Geometry: see drawing. Coordinates: mm, zero at the bounding-box minimum. Coordinates: 2 decimals unless noted, no trailing zeros. Loops run counter-clockwise (first coordinate to the right, second up) from the corner with the lowest first, then second, coordinate; pieces in that order, holes last. Notation, with made-up numbers: (-21.5, 53) -> (-4.5, 53) arc R27 ccw to (-4.5, 70) -> close; hole circle Ø7 at (45.25, 3.5). An arc over 180 degrees is marked (long way). One line per item, written item: value. Start each with the question number.
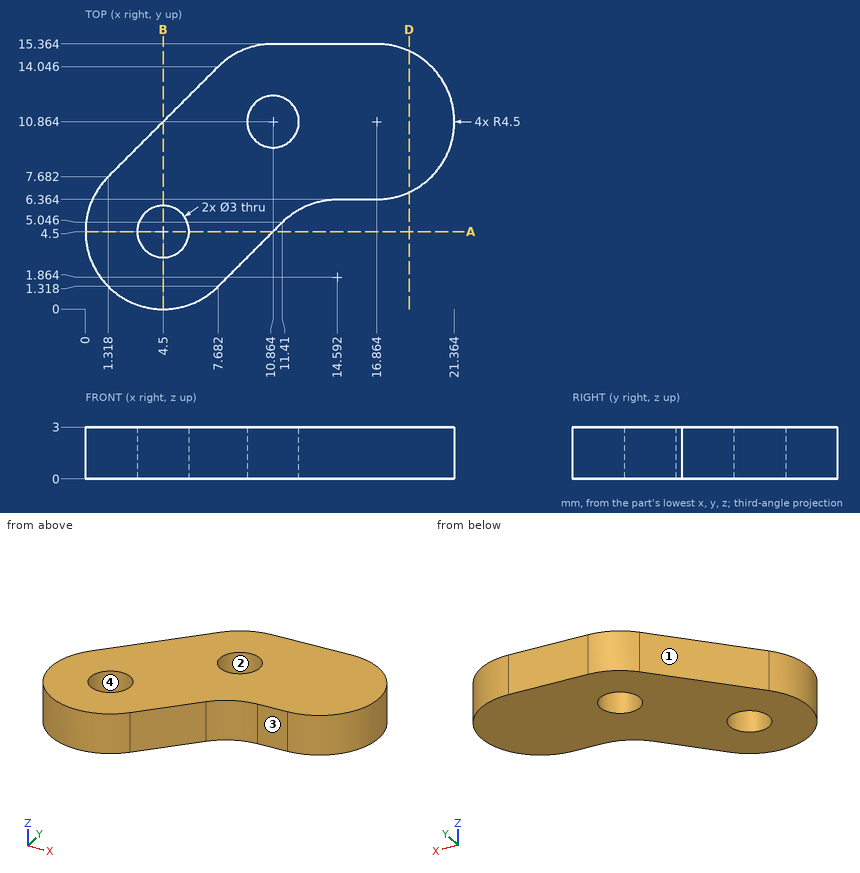
1. Draft query along Y for the marked faces 1, 2, 3 and 4. Return one class per face: released by +Y, released by -Y, zero draft, split by the parting line, or undercut.
2. Section A-A on y = 4.5. Return the cut outline in (x, z), plus the area to 3 significant figures.
3. Section D-D on x = 18.75. Return the cut outline in (y, z), plus the area to 3 significant figures.
4. Pin query (flat end, axial travel): pin 1 Ø1.1 at (x, z) = (16, 1.5) entering from -Y; pin 2 Ø1 at (x, z) = (8.5, 1) entering from +Y. Return the tip coordinate at first contact, or that it passes through.
5. Line query: L1, parallel to Y at x = 4.5, z = 2.25; L2, parallel to X at y = 3.75, z = 0.9; L3, parallel to X at y = 4, z = 0.7. Output: solid intervals per line, ascending. Write a range as [from, to].
Checks:
1. face 1: released by +Y
1. face 2: undercut
1. face 3: released by -Y
1. face 4: undercut
2. outline: (0, 0) -> (3, 0) -> (3, 3) -> (0, 3) -> close; (6, 0) -> (10.86, 0) -> (10.86, 3) -> (6, 3) -> close
2. area: 23.6 mm²
3. outline: (6.78, 0) -> (14.95, 0) -> (14.95, 3) -> (6.78, 3) -> close
3. area: 24.5 mm²
4. pin 1: y = 6.36
4. pin 2: y = 14.96
5. L1: [0, 3], [6, 10.86]
5. L2: [0.06, 3.2], [5.8, 10.11]
5. L3: [0.03, 3.09], [5.91, 10.36]
